from build123d import *

# Parameters (mm, degrees)
SKETCH1_W                 = 152.4
SKETCH1_H                 = 152.4
BOSS_EXTRUDE2_DEPTH       = 25.4
SKETCH2_W                 = 9.652
SKETCH2_H                 = 9.652
BOSS_EXTRUDE3_DEPTH       = 38.1
SKETCH3_W                 = 5.08
SKETCH3_H                 = 3.048
BOSS_EXTRUDE4_DEPTH       = 127
CHAMFER1_SIZE             = 0.508
CHAMFER1_SIZE2            = 0.03552282
CHAMFER2_SIZE             = 0.508
CHAMFER2_SIZE2            = 0.03552282
SKETCH4_W                 = 5.334
SKETCH4_H                 = 3.175
CUT_EXTRUDE3_DEPTH        = 149.86
SKETCH5_R                 = 4.445
BOSS_EXTRUDE5_DEPTH       = 15
F_2_0MM_DOWEL_HOLE1_D     = 2
F_2_0MM_DOWEL_HOLE1_DEPTH = 4.572
F_2_0MM_DOWEL_HOLE1_TIP   = 0.600860619
SHELL1_START              = 2.54
SHELL1_OUTLINE_W          = 147.32
SHELL1_OUTLINE_H          = 141.986
SHELL1_DEPTH              = 20.32
SHELL1_2_OUTLINE_W        = 147.32
SHELL1_2_OUTLINE_H        = 5.334
SHELL1_2_DEPTH            = 6.0325
SHELL1_START_2            = 16.8275
SHELL1_3_OUTLINE_W        = 147.32
SHELL1_3_OUTLINE_H        = 5.334
SHELL1_3_DEPTH            = 6.0325
SHELL1_START_3            = 22.86
SHELL1_4_OUTLINE_W        = 4.572
SHELL1_4_OUTLINE_H        = 4.572
SHELL1_4_DEPTH            = 38.1
SHELL1_START_4            = -6.863890452
SHELL1_5_OUTLINE_R        = 1.905
SHELL1_5_DEPTH            = 9.403890452
SKETCH8_W                 = 19.9
SKETCH8_H                 = 19.9
CUT_EXTRUDE4_DEPTH        = 25.4


with BuildPart() as part:
    # Sketch1 → Boss-Extrude2 (new body)
    with BuildSketch(Plane(origin=(0, 0, 0), x_dir=(1, 0, 0), z_dir=(0, 1, 0))):
        with Locations((53.878787879, -60.325)):
            Rectangle(SKETCH1_W, SKETCH1_H)
    extrude(amount=BOSS_EXTRUDE2_DEPTH)

    # Sketch2 → Boss-Extrude3 (add)
    with BuildSketch(Plane(origin=(0, 25.4, 0), x_dir=(1, 0, 0), z_dir=(0, 1, 0))):
        with Locations((-17.495212121, -131.699)):
            Rectangle(SKETCH2_W, SKETCH2_H)
    extrude(amount=BOSS_EXTRUDE3_DEPTH)

    # Sketch3 → Boss-Extrude4 (add)
    with BuildSketch(Plane.XY.offset(136.525)):
        with Locations((132.618787879, 12.7)):
            Rectangle(SKETCH3_W, SKETCH3_H)
    extrude(amount=-BOSS_EXTRUDE4_DEPTH)

    # Chamfer1
    chamfer1_edges = [part.edges().sort_by_distance(p)[0] for p in [
        (135.158787879, 14.224, 73.025),
    ]]
    chamfer1_side = [part.faces().sort_by_distance(p)[0] for p in [
        (132.618787879, 14.224, 73.025),
    ]]
    chamfer(chamfer1_edges, length=CHAMFER1_SIZE, length2=CHAMFER1_SIZE2, reference=chamfer1_side[0])

    # Chamfer2
    chamfer2_edges = [part.edges().sort_by_distance(p)[0] for p in [
        (135.158787879, 11.176, 73.025),
    ]]
    chamfer2_side = [part.faces().sort_by_distance(p)[0] for p in [
        (132.618787879, 11.176, 73.025),
    ]]
    chamfer(chamfer2_edges, length=CHAMFER2_SIZE, length2=CHAMFER2_SIZE2, reference=chamfer2_side[0])

    # Sketch4 → Cut-Extrude3 (cut)
    with BuildSketch(Plane.ZY.offset(22.321212121)):
        with Locations((-13.208, 12.7)):
            Rectangle(SKETCH4_W, SKETCH4_H)
    extrude(amount=-CUT_EXTRUDE3_DEPTH, mode=Mode.SUBTRACT)

    # Sketch5 → Boss-Extrude5 (add)
    with BuildSketch(Plane(origin=(0, 0, 0), x_dir=(1, 0, 0), z_dir=(0, 1, 0))):
        with Locations(Location((104.578787879, -9.625, 0), (0, 0, 270))):
            Circle(SKETCH5_R)
    extrude(amount=-BOSS_EXTRUDE5_DEPTH)

    # Ø2.0mm Dowel Hole1
    with Locations(Plane(origin=(0, -15, 0), x_dir=(-1, 0, 0), z_dir=(0, -1, 0))):
        with Locations((-104.578787879, -9.625)):
            Hole(F_2_0MM_DOWEL_HOLE1_D / 2, depth=F_2_0MM_DOWEL_HOLE1_DEPTH)
            with Locations((0, 0, -(F_2_0MM_DOWEL_HOLE1_DEPTH + F_2_0MM_DOWEL_HOLE1_TIP / 2))):  # 118° drill point
                Cone(0, F_2_0MM_DOWEL_HOLE1_D / 2, F_2_0MM_DOWEL_HOLE1_TIP, mode=Mode.SUBTRACT)

    # Shell1: read off the stored shape, not the designer's step
    # Shell1 outline → Shell1 (cut)
    with BuildSketch(Plane(origin=(0, 0, 0), x_dir=(1, 0, 0), z_dir=(0, 1, 0)).offset(SHELL1_START)):
        with Locations((53.878787879, -62.992)):
            Rectangle(SHELL1_OUTLINE_W, SHELL1_OUTLINE_H)
    extrude(amount=SHELL1_DEPTH, mode=Mode.SUBTRACT)

    # Shell1 2 outline → Shell1 2 (cut)
    with BuildSketch(Plane(origin=(0, 0, 0), x_dir=(1, 0, 0), z_dir=(0, 1, 0)).offset(SHELL1_START)):
        with Locations((53.878787879, 10.668)):
            Rectangle(SHELL1_2_OUTLINE_W, SHELL1_2_OUTLINE_H)
    extrude(amount=SHELL1_2_DEPTH, mode=Mode.SUBTRACT)

    # Shell1 3 outline → Shell1 3 (cut)
    with BuildSketch(Plane(origin=(0, 0, 0), x_dir=(1, 0, 0), z_dir=(0, 1, 0)).offset(SHELL1_START_2)):
        with Locations((53.878787879, 10.668)):
            Rectangle(SHELL1_3_OUTLINE_W, SHELL1_3_OUTLINE_H)
    extrude(amount=SHELL1_3_DEPTH, mode=Mode.SUBTRACT)

    # Shell1 4 outline → Shell1 4 (cut)
    with BuildSketch(Plane(origin=(0, 0, 0), x_dir=(1, 0, 0), z_dir=(0, 1, 0)).offset(SHELL1_START_3)):
        with Locations((-17.495212121, -131.699)):
            Rectangle(SHELL1_4_OUTLINE_W, SHELL1_4_OUTLINE_H)
    extrude(amount=SHELL1_4_DEPTH, mode=Mode.SUBTRACT)

    # Shell1 5 outline → Shell1 5 (cut)
    with BuildSketch(Plane(origin=(0, 0, 0), x_dir=(1, 0, 0), z_dir=(0, 1, 0)).offset(SHELL1_START_4)):
        with Locations((104.578787879, -9.625)):
            Circle(SHELL1_5_OUTLINE_R)
    extrude(amount=SHELL1_5_DEPTH, mode=Mode.SUBTRACT)

    # Shell1 6 outline → Shell1 6 (revolve, cut)
    with BuildSketch(Plane(origin=(104.578787879, 0, 9.625), x_dir=(1, 0, 0), z_dir=(0, 0, 1))):
        Polygon((0, -6.863890552), (1.905, -8.008530031), (1.905, -6.863890452), align=None)
    revolve(axis=Axis((104.578787879, 0, 9.625), (0, 1, 0)), mode=Mode.SUBTRACT)

    # Sketch8 → Cut-Extrude4 (cut)
    with BuildSketch(Plane.XZ):
        with Locations((120.128787879, -5.925)):
            Rectangle(SKETCH8_W, SKETCH8_H)
    extrude(amount=-CUT_EXTRUDE4_DEPTH, mode=Mode.SUBTRACT)


solid = part.part
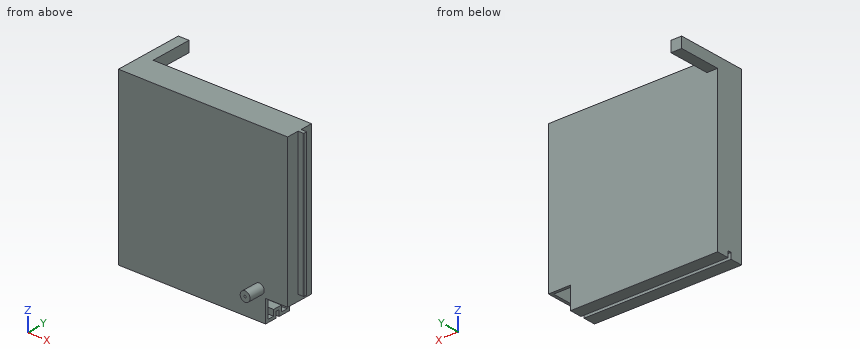
Geometry: final body of the model. Coordinates: model frame, mm. Round coordinates to 2 decimals unless told otherwise and drop trailing zeros. Loops run counter-clockwise (first coordinate to the right, second up) from the corner with the lowest first, then second, coordinate; pieces in that order, holes last. Notation, with made-up numbers: (34.25, -15) - (42.25, -15) arc R16 ccw to (42.25, -1) - close; hole circle Ø7 at (40, 6.5). An arc over 180 degrees is marked (long way). Write each question's results on one line, items separated by ' | '. Start each with the question number.
1) Cut plane A-A on z = -0.5. Return loops of the section in (x, y).
2) Line query: probe 1 along Y at (x, z) = (-1, 129); probe 2 along Z at (x, y) = (62, 18) (3 decimals); probe 3 along X at (y, z) = (12, 127). Output: solid intervals per line, ascending. Write a range as [from, to].
3) Cut plane D-D on z = 109. Return loops of the section in (x, y).
4) Cut plane B-B on y = 37. Return loops of the section in (x, z) (3 decimals), then the cut area to 3 significant figures.
5) Cut plane C-C on x = 33.5. Return loops of the section in (y, z) (1 decimal).
6) First-contact query: P1, Ø4.5, axis at x = 26, z = -11, coming from the +Y side; P2, Ø1.2, axis at x = 104.58, z = 9.62, coming from the -Y side; P3, Ø6, axis at y = 30.5, z = 107, coming from the -X side; P4, Ø1.4, axis at x = -17, z = 132, coming from the -Y side. Flat tips, straight axial feed; report the tip coordinate or a pass-through.
Verdict:
1) outline: (-22.32, 0) - (110.18, 0) - (110.18, 2.54) - (-19.78, 2.54) - (-19.78, 22.86) - (110.18, 22.86) - (110.18, 25.4) - (-22.32, 25.4) - close
2) probe 1: y = [0, 2.54], [22.86, 25.4] | probe 2: z = [-15.875, -13.335], [133.985, 136.525] | probe 3: x = [-22.32, -19.78], [127.54, 135.16]
3) outline: (-22.32, 0) - (130.08, 0) - (130.08, 11.18) - (134.65, 11.18) - (135.16, 11.21) - (135.16, 14.19) - (134.65, 14.22) - (130.08, 14.22) - (130.08, 25.4) - (-22.32, 25.4) - close; hole (-19.78, 2.54) - (127.54, 2.54) - (127.54, 22.86) - (-19.78, 22.86) - close
4) outline: (-22.321, 126.873) - (-12.669, 126.873) - (-12.669, 136.525) - (-22.321, 136.525) - close; hole (-19.781, 129.413) - (-15.209, 129.413) - (-15.209, 133.985) - (-19.781, 133.985) - close | area: 72.3 mm2
5) outline: (0, -15.9) - (11.1, -15.9) - (11.1, -10.5) - (14.3, -10.5) - (14.3, -15.9) - (25.4, -15.9) - (25.4, 136.5) - (0, 136.5) - close; hole (2.5, -13.3) - (8.6, -13.3) - (8.6, -8) - (16.8, -8) - (16.8, -13.3) - (22.9, -13.3) - (22.9, 134) - (2.5, 134) - close
6) P1: stops at y = 25.4 | P2: stops at y = -10.19 | P3: passes through | P4: stops at y = 0
